Geometry check sheet. Reference: the model listing, model coordinates, mm. Give positions to 0.01 mm unless a question says otherwise; leave off trailing zeros. Use a Markdown table: item, result.
```python
from build123d import *

# Parameters (mm, degrees)
SKETCH001002010_W         = 401
SKETCH001002010_H         = 44
SKETCH001002010_R         = 1.5
SKETCH001002010_R_2       = 15
SKETCH001002010_R_3       = 10
SKETCH001002010_W_2       = 3
SKETCH001002010_H_2       = 9.8
SKETCH001002010_W_3       = 9.8
SKETCH001002010_H_3       = 3
PAD015_DEPTH              = 3
POCKET009_DEPTH           = 3
SKETCH001002027_R         = 2.5
POCKET010_DEPTH           = 3
FILLET028_R               = 5
FILLET028_PLACEMENT_ANGLE = 90


with BuildPart() as part:
    # Sketch001002010 → Pad015 (new body)
    with BuildSketch(Plane.XZ.offset(-106)):
        Rectangle(SKETCH001002010_W, SKETCH001002010_H)
        with Locations((-194, 0)):
            Circle(SKETCH001002010_R, mode=Mode.SUBTRACT)
        with Locations((194, 0)):
            Circle(SKETCH001002010_R, mode=Mode.SUBTRACT)
        with Locations((-121.5, 0)):
            Circle(SKETCH001002010_R_2, mode=Mode.SUBTRACT)
        with Locations((-146.5, 10)):
            Circle(SKETCH001002010_R, mode=Mode.SUBTRACT)
        with Locations((-186.5, -10)):
            Circle(SKETCH001002010_R, mode=Mode.SUBTRACT)
        with Locations((87.5, -10)):
            Circle(SKETCH001002010_R, mode=Mode.SUBTRACT)
        with Locations((147.5, 10)):
            Circle(SKETCH001002010_R, mode=Mode.SUBTRACT)
        with Locations((-38, 0)):
            Circle(SKETCH001002010_R, mode=Mode.SUBTRACT)
        with Locations((-96.5, -10)):
            Circle(SKETCH001002010_R, mode=Mode.SUBTRACT)
        with Locations((-46.5, 10)):
            Circle(SKETCH001002010_R, mode=Mode.SUBTRACT)
        with Locations((62.5, 0)):
            Circle(SKETCH001002010_R_3, mode=Mode.SUBTRACT)
        with Locations((194, 9.1)):
            Rectangle(SKETCH001002010_W_2, SKETCH001002010_H_2, mode=Mode.SUBTRACT)
        with Locations((194, -9.1)):
            Rectangle(SKETCH001002010_W_2, SKETCH001002010_H_2, mode=Mode.SUBTRACT)
        with Locations((-194, 9.1)):
            Rectangle(SKETCH001002010_W_2, SKETCH001002010_H_2, mode=Mode.SUBTRACT)
        with Locations((-194, -9.1)):
            Rectangle(SKETCH001002010_W_2, SKETCH001002010_H_2, mode=Mode.SUBTRACT)
        with Locations((-173.5, -18)):
            Rectangle(SKETCH001002010_W_3, SKETCH001002010_H_3, mode=Mode.SUBTRACT)
        with Locations((93.5, -18)):
            Rectangle(SKETCH001002010_W_3, SKETCH001002010_H_3, mode=Mode.SUBTRACT)
        with Locations((-173.5, 19)):
            Rectangle(SKETCH001002010_W_3, SKETCH001002010_H_3, mode=Mode.SUBTRACT)
        with Locations((93.5, 19)):
            Rectangle(SKETCH001002010_W_3, SKETCH001002010_H_3, mode=Mode.SUBTRACT)
        with Locations((-38, 9.1)):
            Rectangle(SKETCH001002010_W_2, SKETCH001002010_H_2, mode=Mode.SUBTRACT)
        with Locations((-38, -9.1)):
            Rectangle(SKETCH001002010_W_2, SKETCH001002010_H_2, mode=Mode.SUBTRACT)
    extrude(amount=-PAD015_DEPTH)

    # Sketch001002026 → Pocket009 (cut)
    with BuildSketch(Plane.XZ.offset(-106)):
        with BuildLine():
            Line((-17, 3.05), (-17, -11.05))
            ThreePointArc((-17, -11.05), (-16.414214, -12.464214), (-15, -13.05))
            Line((-15, -13.05), (34.6, -13.05))
            ThreePointArc((34.6, -13.05), (36.014214, -12.464214), (36.6, -11.05))
            Line((36.6, -11.05), (36.6, 3.05))
            ThreePointArc((36.6, 3.05), (36.014214, 4.464214), (34.6, 5.05))
            Line((34.6, 5.05), (-15, 5.05))
            ThreePointArc((-15, 5.05), (-16.414214, 4.464214), (-17, 3.05))
        make_face()
    extrude(amount=-POCKET009_DEPTH, mode=Mode.SUBTRACT)

    # Sketch001002027 → Pocket010 (cut)
    with BuildSketch(Plane(origin=(0, 109, 0), x_dir=(-1, 0, 0), z_dir=(0, 1, 0))):
        with Locations((-179.85, 11.5)):
            Circle(SKETCH001002027_R)
        with Locations((-179.85, -11.5)):
            Circle(SKETCH001002027_R)
        with BuildLine():
            Line((-185.35, 7), (-185.35, -4.5))
            ThreePointArc((-185.35, -4.5), (-185.057107, -5.207107), (-184.35, -5.5))
            Line((-184.35, -5.5), (-175.35, -5.5))
            ThreePointArc((-175.35, -5.5), (-174.642893, -5.207107), (-174.35, -4.5))
            Line((-174.35, -4.5), (-174.35, 4.5))
            ThreePointArc((-174.35, 4.5), (-174.642893, 5.207107), (-175.35, 5.5))
            Line((-175.35, 5.5), (-181.35, 5.5))
            ThreePointArc((-182.85, 7), (-182.41066, 5.93934), (-181.35, 5.5))
            ThreePointArc((-182.85, 7), (-184.1, 8.25), (-185.35, 7))
        make_face()
        with BuildLine():
            Line((-169.85, 3), (-169.85, -11))
            ThreePointArc((-169.85, -11), (-169.557107, -11.707107), (-168.85, -12))
            Line((-168.85, -12), (-158.85, -12))
            ThreePointArc((-158.85, -12), (-158.142893, -11.707107), (-157.85, -11))
            Line((-157.85, -11), (-157.85, 3))
            ThreePointArc((-157.85, 3), (-158.142893, 3.707107), (-158.85, 4))
            Line((-158.85, 4), (-168.85, 4))
            ThreePointArc((-168.85, 4), (-169.557107, 3.707107), (-169.85, 3))
        make_face()
    extrude(amount=-POCKET010_DEPTH, mode=Mode.SUBTRACT)

    # Fillet028
    fillet028_edges = [part.edges().sort_by_distance(p)[0] for p in [
        (-200.5, 107.5, 22),
        (200.5, 107.5, 22),
        (-200.5, 107.5, -22),
        (200.5, 107.5, -22),
    ]]
    fillet(fillet028_edges, radius=FILLET028_R)


with BuildPart() as part_1:
    # Fillet028 placement: moved
    add(part.part.rotate(Axis((0, 0, 0), (-1, 0, 0)), FILLET028_PLACEMENT_ANGLE))


solid = part_1.part
```
1) Material ranges on L1, parallel to Y at x = 194, z = -107.7; L2, parallel to Y at x = -1, z = -106.85; L3, parallel to Y at x = 179.85, z = -107, recorded low to high. Write a range as from..to.
Working result:
| item | result |
|---|---|
| L1 | y = -22..-14, -4.2..-1.5, 1.5..4.2, 14..22 |
| L2 | y = -22..-13.05, 5.05..22 |
| L3 | y = -22..-14, -9..-5.5, 5.5..9, 14..22 |
2) Depth check by flat-ended pin: P1, Ø0.9, axis at y = -18, z = -107, coming from the +X side; P2, Ø0.9, axis at y = 18.5, z = -107.5, coming from the -X side; P3, Ø1.5, axis at y = 19, z = -107, coming from the +X side. Enter the tip coordinate at first touch or a pass-through.
Working result:
| item | result |
|---|---|
| P1 | stops at x = 200.47 |
| P2 | stops at x = -200.39 |
| P3 | stops at x = 200.34 |
3) Section check A-A on z = -106.8. Count the separate pieces of the cut face and the enclosed holes in it, then the cut area to 3 significant figures.
Working result:
| item | result |
|---|---|
| separate pieces | 1 |
| enclosed holes | 26 |
| area | 14,900 mm² |
4) Mould release check, pull along X, two halves, no side actions. Record for faces 1 (the flat face through (-3, 10, -109)), 2 (the cylindrical face through (-136.485, 0.66, -107.479)): pulls with the +X half, pulls with the -X half, needs draft (parallel to the pull), parting line crosses it, or undercut.
Working result:
| item | result |
|---|---|
| face 1 | needs draft |
| face 2 | undercut |
